Solid Edge part; units mm, degrees
sketch "Sketch1" plane through (0, 0, 0) normal (0, 0, 1) x (1, 0, 0)
  line L0 (-6.1009, 4.0673) -> (-6.5728, -3.2499)
  line L1 (-6.5728, -3.2499) -> (-0.4719, -7.3171)
  line L2 (-0.4719, -7.3171) -> (6.1009, -4.0673)
  line L3 (6.1009, -4.0673) -> (6.5728, 3.2499)
  line L4 (6.5728, 3.2499) -> (0.4719, 7.3171)
  line L5 (0.4719, 7.3171) -> (-6.1009, 4.0673)
extrude "Protrusion1" add sketch "Sketch1" against normal blind 575
sketch "Sketch2" plane through (0, 0, -2) normal (0, 0, 1) x (-0.8964, -0.4432, 0)
  circle A0 centre (0, 0) radius 5.5
  circle A1 centre (0, 0) radius 13.1424
extrude "ExtrudedCutout_1" cut sketch "Sketch2" against normal blind 2
sketch "Sketch3" plane through (0, 0, -573) normal (0, 0, -1) x (0.8964, 0.4432, 0)
  circle A0 centre (0, 0) radius 5.5
  circle A1 centre (0, 0) radius 13.1424
extrude "ExtrudedCutout_2" cut sketch "Sketch3" against normal blind 2
properties part number "BumbleB0544"
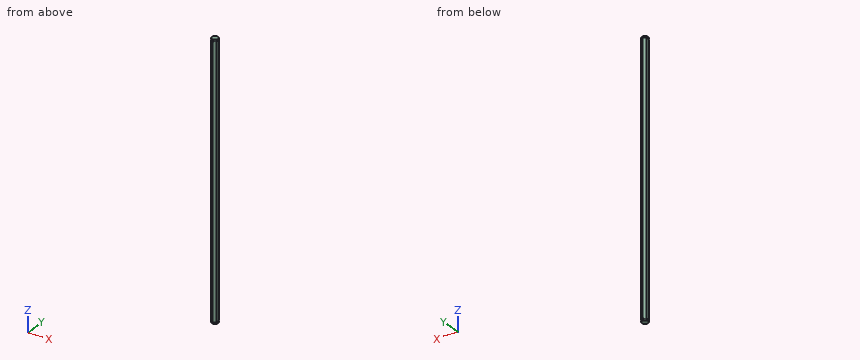
Can you work these out from the model? Positions are in its coordinate system, mm. Give positions to 0.01 mm unless a question says otherwise; leave off trailing zeros. Order: outer loops, then holes, each group sorted by start corner. A loop starts at its lowest first (then second) coordinate and runs counter-clockwise, first axis right, second up. Notation, with made-up numbers: M 18.25,63 L 73.25,63 A25 ccw 73.25,80 Z; hole C -31,40 d7. An arc over 180 degrees is marked long. One line per item, written item: value.
1) I want a section at A-A, the plane y = 0. List the corners of the cut face in (x, z) for me, plus the area to 3 significant figures.
Answer sheet:
outline: M -6.36,-575 L 6.36,-575 L 6.36,-573 L 5.5,-573 L 5.5,-571 L 6.36,-571 L 6.36,-4 L 5.5,-4 L 5.5,-2 L 6.36,-2 L 6.36,0 L -6.36,0 L -6.36,-2 L -5.5,-2 L -5.5,-4 L -6.36,-4 L -6.36,-571 L -5.5,-571 L -5.5,-573 L -6.36,-573 Z
area: 7,310 mm^2
2) Please list where these lines run through material, in increasing order: line 1 along Z through (x, y) = (-5.75, 2.5); line 2 along Y through (x, z) = (-3.25, -270.5); line 3 along X through (y, z) = (-2.75, -319).
Answer sheet:
line 1: z = -575 to -573, -571 to -4, -2 to 0
line 2: y = -5.47 to 5.48
line 3: x = -6.54 to 6.19
3) I want a section at B-B, the plane z = -187.5. List the corners of the cut face in (x, y) for me.
Answer sheet:
outline: M -6.57,-3.25 L -0.47,-7.32 L 6.1,-4.07 L 6.57,3.25 L 0.47,7.32 L -6.1,4.07 Z
4) For P1, Ø1, axis at x = 3, z = -243.5, coming from the -Y side, with a flat end and sliding along its axis, tell me the tip position at first contact or that it passes through.
Answer sheet:
P1: stops at y = -5.85
